Geometry: final body of the model. Coordinates: model frame, mm. A direction names the side the tool comes from. Give positions to 0.01 mm unless a question says otherwise; leave off trailing zeros. Write each loop counter-clockwise with the first axis right and the second up, starting at its lowest first coordinate (ties: lowest second). Pieces come first, ordered by that corner, then holes.
from build123d import *

# Parameters (mm, degrees)
SKETCH2_W           = 15
SKETCH2_H           = 30
SKETCH2_W_2         = 30
SKETCH2_H_2         = 15
CUT_EXTRUDE1_DEPTH  = 5
SKETCH3_W           = 29.529404499
SKETCH3_H           = 3.5
SKETCH3_W_2         = 3.5
SKETCH3_H_2         = 29.529404499
BOSS_EXTRUDE1_DEPTH = 2


with BuildPart() as part:
    # Sketch1 → Revolve2 (revolve)
    with BuildSketch(Plane.XY):
        Polygon((0, 4), (0, 60), (-10, 60), (-10, 15), (-25, 15), (-25, 4), align=None)
    revolve(axis=Axis((0, 0, 0), (-1, 0, 0)))

    # Sketch2 → Cut-Extrude1 (cut)
    with BuildSketch(Plane(origin=(0, 0, 0), x_dir=(0, 0, -1), z_dir=(1, 0, 0))):
        Polygon((15.909902577, 26.516504294), (37.123106012, 47.72970773), (47.72970773, 37.123106012), (26.516504294, 15.909902577), align=None)
        with Locations((0, 45)):
            Rectangle(SKETCH2_W, SKETCH2_H)
        with Locations((45, 0)):
            Rectangle(SKETCH2_W_2, SKETCH2_H_2)
        Polygon((26.516504295, -15.909902577), (47.72970773, -37.123106012), (37.123106012, -47.72970773), (15.909902577, -26.516504294), align=None)
        with Locations((0, -45)):
            Rectangle(SKETCH2_W, SKETCH2_H)
        Polygon((-15.909902577, -26.516504294), (-37.123106012, -47.72970773), (-47.72970773, -37.123106012), (-26.516504294, -15.909902577), align=None)
        with Locations((-45, 0)):
            Rectangle(SKETCH2_W_2, SKETCH2_H_2)
        Polygon((-26.516504294, 15.909902577), (-47.72970773, 37.123106012), (-37.123106012, 47.72970773), (-15.909902577, 26.516504294), align=None)
    extrude(amount=-CUT_EXTRUDE1_DEPTH, mode=Mode.SUBTRACT)

    # Sketch3 → Boss-Extrude1 (add)
    with BuildSketch(Plane(origin=(0, 0, 0), x_dir=(0, 0, -1), z_dir=(1, 0, 0))):
        Polygon((-15.909902577, 26.516504294), (-36.790344742, 47.39694646), (-39.265218476, 44.922072726), (-18.384776311, 24.04163056), align=None)
        Polygon((-24.04163056, 18.384776311), (-44.922072726, 39.265218476), (-47.39694646, 36.790344742), (-26.516504294, 15.909902577), align=None)
        with Locations((-44.76470225, 5.75)):
            Rectangle(SKETCH3_W, SKETCH3_H)
        with Locations((-44.76470225, -5.75)):
            Rectangle(SKETCH3_W, SKETCH3_H)
        Polygon((-26.516504294, -15.909902577), (-47.39694646, -36.790344742), (-44.922072726, -39.265218476), (-24.04163056, -18.384776311), align=None)
        Polygon((-18.384776311, -24.04163056), (-39.265218476, -44.922072726), (-36.790344742, -47.39694646), (-15.909902577, -26.516504294), align=None)
        with Locations((-5.75, -44.76470225)):
            Rectangle(SKETCH3_W_2, SKETCH3_H_2)
        with Locations((5.75, -44.76470225)):
            Rectangle(SKETCH3_W_2, SKETCH3_H_2)
        Polygon((36.790344742, -47.39694646), (39.265218476, -44.922072726), (18.384776311, -24.04163056), (15.909902577, -26.516504294), align=None)
        Polygon((44.922072726, -39.265218476), (47.39694646, -36.790344742), (26.516504295, -15.909902577), (24.04163056, -18.384776311), align=None)
        with Locations((44.76470225, -5.75)):
            Rectangle(SKETCH3_W, SKETCH3_H)
        with Locations((44.76470225, 5.75)):
            Rectangle(SKETCH3_W, SKETCH3_H)
        Polygon((47.39694646, 36.790344742), (44.922072726, 39.265218476), (24.04163056, 18.384776311), (26.516504294, 15.909902577), align=None)
        Polygon((39.265218476, 44.922072726), (36.790344742, 47.39694646), (15.909902577, 26.516504294), (18.384776311, 24.04163056), align=None)
        with Locations((5.75, 44.76470225)):
            Rectangle(SKETCH3_W_2, SKETCH3_H_2)
        with Locations((-5.75, 44.76470225)):
            Rectangle(SKETCH3_W_2, SKETCH3_H_2)
    extrude(amount=-BOSS_EXTRUDE1_DEPTH)


solid = part.part
Q1. Section C-C on x = -18.5. Output: boundary loops of the cut face in (y, z), plus the area to 3 significant figures.
Filled sheet:
outline: circle Ø30 at (0, 0); hole circle Ø8 at (0, 0)
area: 657 mm2
Q2. Ray query, line 1 along Z through (x, y) = (-19.75, 0); line 2 along Y through (x, z) = (-8.5, 0). Return the intervals inside material, ascending.
Filled sheet:
line 1: z = -15 to -4, 4 to 15
line 2: y = -60 to -4, 4 to 60
Q3. Section A-A on y = 0. Output: boundary loops of the cut face in (x, z), plus the area to 3 significant figures.
Filled sheet:
outline: (-25, -15) - (-10, -15) - (-10, -60) - (-5, -60) - (-5, -30) - (0, -30) - (0, -4) - (-25, -4) - close; (-25, 4) - (0, 4) - (0, 30) - (-5, 30) - (-5, 60) - (-10, 60) - (-10, 15) - (-25, 15) - close
area: 1,150 mm2
Q4. Pull-direction query (Z, two-part tool) for faces 1 (the flat face through (-0.986, -28.971, 34.628)), 2 (the flat face through (-2, 6, 45)); classes: released by +Z, released by -Z, zero draft, split by the parting line, or undercut.
Filled sheet:
face 1: undercut
face 2: zero draft
Q5. Pin query (flat end, axial travel): P1, Ø15.5, axis at y = 25, z = -37, coming from the +X side; P2, Ø0.6, axis at x = -0.5, z = -51.5, coming from the +Y side; P3, Ø4, axis at x = -9.5, y = 20, coming from the -Z side; P4, Ø5, axis at x = -17, z = 5, coming from the -Y side. Return the tip coordinate at first contact, or that it passes through.
Filled sheet:
P1: stops at x = 0
P2: stops at y = 31.28
P3: stops at z = -57.24
P4: stops at y = -14.79
Q6. Access query for faces 3 (the flat face through (-2, 45, -6)), 4 (the flat face through (-0.986, 28.679, 34.336)), 5 (the flat face through (-3.021, 21.139, -21.287)), 6 (the flat face through (-10, 12, 12)). Directions: +Z, -Z, +X, -X, +Y, -Y. A direction counts if a zero-diameter tool reaches every point of the face in a straight line with its end or side. Return the directions, or none.
Filled sheet:
face 3: +Y
face 4: +X
face 5: none
face 6: -X
Q7. Section D-D on z = 53. Output: boundary loops of the cut face in (x, y), plus the area to 3 significant figures.
Filled sheet:
outline: (-10, -28.12) - (0, -28.12) - (0, -4) - (-2, -4) - (-2, -7.5) - (-5, -7.5) - (-5, 7.5) - (-2, 7.5) - (-2, 4) - (0, 4) - (0, 28.12) - (-10, 28.12) - close
area: 501 mm2
